from build123d import *

# Parameters (mm, degrees)
F0_R     = 2.01
F0_R_2   = 7.5
F1_DEPTH = 5
F2_SIZE  = 3
F3_R     = 11
F4_DEPTH = 3
F5_R     = 17.5
F5_R_2   = 11
F6_DEPTH = 4.2
F7_SIZE  = 4.19999


# Not quite as in the source:
# - a fillet or chamfer is up to 0.001 mm smaller than in the source, because OpenCascade refuses the exact size


with BuildPart() as f1:
    # F0 (on Front) → F1 (new body)
    with BuildSketch(Plane.XZ):
        Polygon((0, 70), (0, 0), (0, -50), (65, -50), (80, -35), (80, 70), align=None)
        with Locations((10, -30)):
            Circle(F0_R, mode=Mode.SUBTRACT)
        with BuildLine():
            ThreePointArc((24.9080765748, -28.5), (26.4180765748, -26.99), (27.9280765748, -28.5))
            Line((27.9280765748, -28.5), (27.9280765748, -32.5))
            ThreePointArc((27.9280765748, -32.5), (26.4180765748, -34.01), (24.9080765748, -32.5))
            Line((24.9080765748, -32.5), (24.9080765748, -28.5))
        make_face(mode=Mode.SUBTRACT)
        with Locations((10, 0)):
            Circle(F0_R, mode=Mode.SUBTRACT)
        with BuildLine():
            ThreePointArc((27.9280765748, -1.5), (26.4180765748, -3.01), (24.9080765748, -1.5))
            Line((24.9080765748, -1.5), (24.9080765748, 2.5))
            ThreePointArc((24.9080765748, 2.5), (26.4180765748, 4.01), (27.9280765748, 2.5))
            Line((27.9280765748, 2.5), (27.9280765748, -1.5))
        make_face(mode=Mode.SUBTRACT)
        with BuildLine():
            ThreePointArc((55.9080765748, -28.5), (57.4180765748, -26.99), (58.9280765748, -28.5))
            Line((58.9280765748, -28.5), (58.9280765748, -32.5))
            ThreePointArc((58.9280765748, -32.5), (57.4180765748, -34.01), (55.9080765748, -32.5))
            Line((55.9080765748, -32.5), (55.9080765748, -28.5))
        make_face(mode=Mode.SUBTRACT)
        with BuildLine():
            ThreePointArc((30.4180765748, -11), (41.9180765748, 0.5), (53.4180765748, -11))
            Line((53.4180765748, -11), (53.4180765748, -19))
            ThreePointArc((53.4180765748, -19), (41.9180765748, -30.5), (30.4180765748, -19))
            Line((30.4180765748, -19), (30.4180765748, -11))
        make_face(mode=Mode.SUBTRACT)
        with BuildLine():
            ThreePointArc((58.9280765748, -1.5), (57.4180765748, -3.01), (55.9080765748, -1.5))
            Line((55.9080765748, -1.5), (55.9080765748, 2.5))
            ThreePointArc((55.9080765748, 2.5), (57.4180765748, 4.01), (58.9280765748, 2.5))
            Line((58.9280765748, 2.5), (58.9280765748, -1.5))
        make_face(mode=Mode.SUBTRACT)
        with Locations((10, 30)):
            Circle(F0_R, mode=Mode.SUBTRACT)
        with Locations((10, 60)):
            Circle(F0_R, mode=Mode.SUBTRACT)
        with Locations((58.25, 25)):
            Circle(F0_R_2, mode=Mode.SUBTRACT)
        with Locations((40, 60)):
            Circle(F0_R, mode=Mode.SUBTRACT)
        with Locations((70, 60)):
            Circle(F0_R, mode=Mode.SUBTRACT)
    extrude(amount=F1_DEPTH)

    # F2
    f2_edges = [f1.edges().sort_by_distance(p)[0] for p in [
        (80, 0, 17.5),
        (40, 0, 70),
        (0, 0, 10),
        (32.5, 0, -50),
        (72.5, 0, -42.5),
    ]]
    chamfer(f2_edges, length=F2_SIZE)

    # F3 (on face) → F4 (cut)
    with BuildSketch(Plane.XZ.offset(5)):
        with Locations((58.25, 25)):
            Circle(F3_R)
    extrude(amount=-F4_DEPTH, mode=Mode.SUBTRACT)

    # F5 (on face) → F6 (join)
    with BuildSketch(Plane.XZ.offset(5)):
        with Locations((58.25, 25)):
            Circle(F5_R)
        with Locations((58.25, 25)):
            Circle(F5_R_2, mode=Mode.SUBTRACT)
    extrude(amount=F6_DEPTH)

    # F7 (size 4.2 in the source; OpenCascade refuses exactly that, so slightly less here)
    f7_edges = [f1.edges().sort_by_distance(p)[0] for p in [
        (40.75, -9.2, 25),
    ]]
    chamfer(f7_edges, length=F7_SIZE)


solid = f1.part
Design review of the part built by this model. Coordinates are the model's own, in mm. A direction names the side the tool comes from. Give positions to 0.01 mm unless a question says otherwise; leave off trailing zeros. Loops run counter-clockwise (first coordinate to the right, second up) from the corner with the lowest first, then second, coordinate; pieces in that order, holes last. Notation, with made-up numbers: (-4.5, 75) - (29.5, 75) arc R32 cw to (29.5, 106) - close; hole circle Ø10 at (73.5, 66). An arc over 180 degrees is marked (long way). Write item = value, one per line.
1) Take a section at D-D on y = -6.25. State the section outline as (x, z) points, and give its area (3 significant figures).
Result sheet:
outline = circle Ø32.5 at (58.25, 25); hole circle Ø22 at (58.25, 25)
area = 449 mm2
2) Take a section at A-A on z = -13. State the section outline as (x, y) points.
Result sheet:
outline = (0, -5) - (30.42, -5) - (30.42, 0) - (3, 0) - (0, -3) - close; (53.42, -5) - (80, -5) - (80, -3) - (77, 0) - (53.42, 0) - close
3) Take a section at C-C on x = 19. State the section outline as (y, z) points.
Result sheet:
outline = (-5, -50) - (-3, -50) - (0, -47) - (0, 67) - (-3, 70) - (-5, 70) - close
4) Clearance check with flat-ended pins moving along their axes: pin 1 Ø3.5 at (x, z) = (10, -30) entering from +Y; pin 2 Ø1.5 at (x, z) = (71, -14) entering from -Y. State where each tip first meets the part, or that it passes through.
Result sheet:
pin_1 = through
pin_2 = -5
5) Tool access review of faces 1 (the face through (57.45, -2.46, -34.01)), 2 (the face through (39, 0, 11)): name each direction out of +Z, -Z, +X, -X, +Y, -Y from which nothing blocks a thin tool from reaching the whole face with its end or side.
Result sheet:
face_1 = +Y, -Y
face_2 = +Z, -Z, +X, -X, +Y
6) Take a section at B-B on z = 60. State the section outline as (x, y) points, and give its area (3 significant figures).
Result sheet:
outline = (0, -5) - (7.99, -5) - (7.99, 0) - (3, 0) - (0, -3) - close; (12.01, -5) - (37.99, -5) - (37.99, 0) - (12.01, 0) - close; (42.01, -5) - (67.99, -5) - (67.99, 0) - (42.01, 0) - close; (72.01, -5) - (80, -5) - (80, -3) - (77, 0) - (72.01, 0) - close
area = 331 mm2
7) To check wall thickness, follow line 1 (Z direction, x = 10, y = -3.7); line 2 (Y direction, x = 5.5, z = 60); line 3 (Z direction, x = 58.5, y = -2.25). State the ranges of each line that lie inside material, in increasing order.
Result sheet:
line_1 = -50 to -32.01, -27.99 to -2.01, 2.01 to 27.99, 32.01 to 57.99, 62.01 to 70
line_2 = -5 to 0
line_3 = -49.25 to -33.55, -27.45 to -2.55, 3.55 to 14, 36 to 69.25
8) Draft analysis for pull direction X (two halves, no side actions). For faces 3 (the face through (49.52, -5.55, 18.31)), 4 (the face through (71.32, -1.48, -41.53)), 5 (the face through (32, -1, -48)), 6 (the face through (57.38, -2.46, 4.01)), state which applies: +X half, -X half, draft (parallel to the pull), parting line (faces both ways), or undercut.
Result sheet:
face_3 = undercut
face_4 = +X half
face_5 = draft
face_6 = undercut
